```python
from build123d import *

# Parameters (mm, degrees)
SKETCH1_W              = 25.4
SKETCH1_H              = 25.4
SKETCH1_W_2            = 19.05
SKETCH1_H_2            = 19.05
EXTRUDE_THIN1_DEPTH    = 660.4
SKETCH4_R              = 9.525
CUT_EXTRUDE1_DEPTH     = 662.376201568
F_10_CLEARANCE_HOLE2_D = 5.1054
F_10_CLEARANCE_HOLE3_D = 5.1054


with BuildPart() as part:
    # Sketch1 → Extrude-Thin1 (new body)
    with BuildSketch(Plane.XY):
        with Locations((-12.7, 12.7)):
            Rectangle(SKETCH1_W, SKETCH1_H)
        with Locations((-12.7, 12.7)):
            Rectangle(SKETCH1_W_2, SKETCH1_H_2, mode=Mode.SUBTRACT)
    extrude(amount=EXTRUDE_THIN1_DEPTH)

    # Sketch4 → Cut-Extrude1 (cut, through all)
    with BuildSketch(Plane.ZY.offset(25.4)):
        with Locations((241.3, 12.7)):
            Circle(SKETCH4_R)
    extrude(amount=-CUT_EXTRUDE1_DEPTH, mode=Mode.SUBTRACT)

    # #10 Clearance Hole2 (through all)
    with Locations(Plane.ZY.offset(25.4)):
        with Locations((12.7, 12.7), (25.4, 12.7), (38.1, 12.7)):
            Hole(F_10_CLEARANCE_HOLE2_D / 2)

    # #10 Clearance Hole3 (through all)
    with Locations(Plane.ZY.offset(25.4)):
        with Locations((622.3, 12.7), (635, 12.7), (647.7, 12.7)):
            Hole(F_10_CLEARANCE_HOLE3_D / 2)


solid = part.part
```
Input: part model. Units: mm. Frame: model coordinates. A direction names the side the tool comes from. Give positions to 0.01 mm unless a question says otherwise; leave off trailing zeros. Order: outer loops, then holes, each group sorted by start corner. A loop starts at its lowest first (then second) coordinate and runs counter-clockwise, first axis right, second up.
1. Reachability of faces 1 (the flat face through (-13, 0, 326)), 2 (the flat face through (-3.175, 13, 448)) from +Z, -Z, +X, -X, +Y, -Y: full face, straight path, thin tool, end or side. Return the list, or none.
Derived:
face 1: +Z, -Z, +X, -X, -Y
face 2: +Z, -Z
2. Mould query, pull axis X, two halves, no side actions, for faces 3 (the flat face through (-22.225, 13, 119)), 4 (the flat face through (-2, 13, 660.4)), 5 (the flat face through (-25.4, 13, 326)). Classes: released by +X, released by -X, zero draft, split by the parting line, or undercut.
Derived:
face 3: undercut
face 4: zero draft
face 5: released by -X
3. Section B-B on z = 145. Return the cut outline in (x, y) (3 decimals).
Derived:
outline: (-25.4, 0) - (0, 0) - (0, 25.4) - (-25.4, 25.4) - close; hole (-22.225, 3.175) - (-3.175, 3.175) - (-3.175, 22.225) - (-22.225, 22.225) - close
4. Pin query (flat end, axial travel): pin 1 (4.5 mm diameter, centred on y = 12.7, z = 647.7, fed in from -X). Return the tip coordinate at first contact, or that it passes through.
Derived:
pin 1: passes through
5. Material intervals for L1, parallel to X at y = 10.25, z = 310 (3 decimals); L2, parallel to Y at x = -11.5, z = 289 (3 decimals); L3, parallel to Y at x = -0.65, z = 647.7, sorted ascending.
Derived:
L1: x = -25.4 to -22.225, -3.175 to 0
L2: y = 0 to 3.175, 22.225 to 25.4
L3: y = 0 to 10.15, 15.25 to 25.4
6. Section A-A on x = -17.25. Return the cut outline in (y, z) (3 decimals).
Derived:
outline: (0, 0) - (3.175, 0) - (3.175, 660.4) - (0, 660.4) - close; (22.225, 0) - (25.4, 0) - (25.4, 660.4) - (22.225, 660.4) - close
